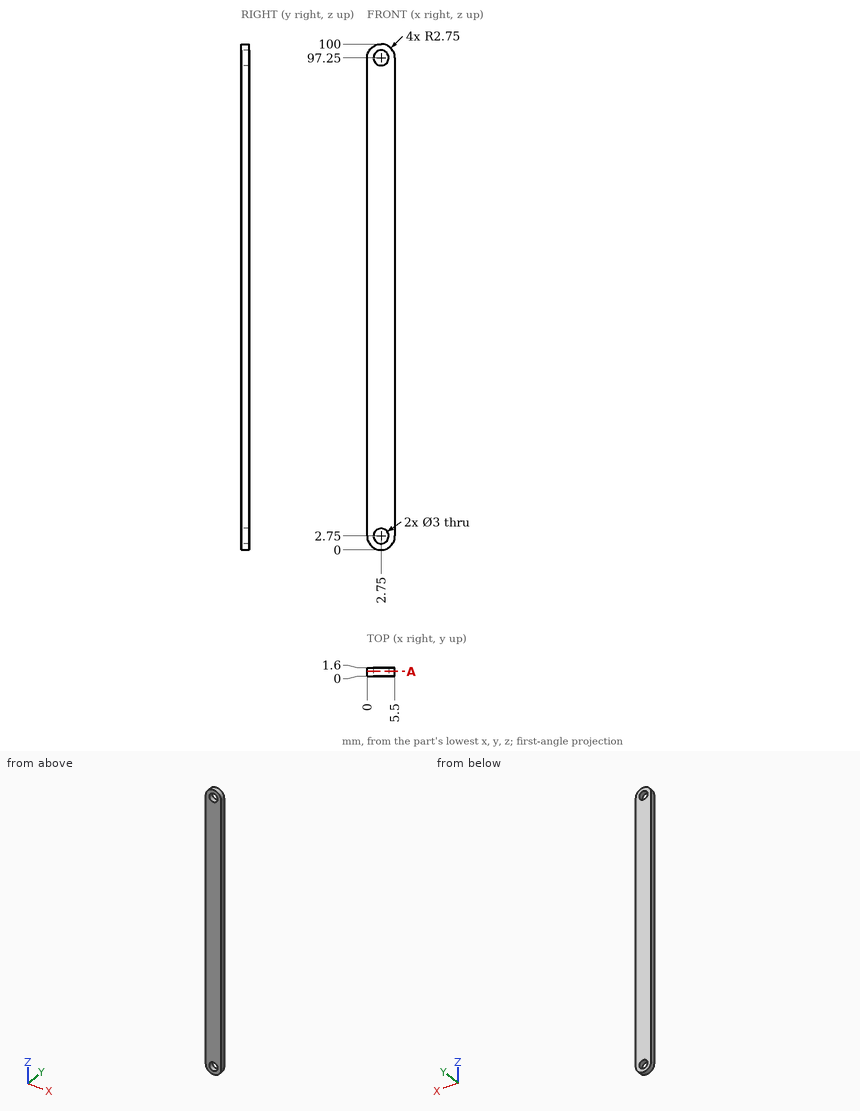
For this review, use the dimensioned drawing (mm, ordinates from the lowest corner) and the shaded views. Give positions to 0.01 mm unless a question says otherwise; leave off trailing zeros. Use one line per item in the form item = value. Start each with the question number.
Item 1: We need section A-A on y = 0.9. Give the number of separate pieces and of enclosed holes in the cut face, plus the area to 3 significant figures.
Item 2: Insertion check: pin 1 Ø2.5 at (x, z) = (2.75, 2.75) entering from -Y. The pin has a flat end and moves straight along its axis. Give the tip position at first contact, or say it passes through.
Item 3: To check wall thickness, follow line 1 along Z through (x, y) = (2.75, 1.1); line 2 along Z through (x, y) = (3.3, 1.15); line 3 along X through (y, z) = (1.2, 97.25). State the ranges of each line that lie inside material, in increasing order. Write a range as from..to.
Completed:
q1.separate_pieces = 1
q1.enclosed_holes = 2
q1.area = 529 mm²
q2.pin_1 = through
q3.line_1 = 0..1.25, 4.25..95.75, 98.75..100
q3.line_2 = 0.06..1.35, 4.15..95.85, 98.65..99.94
q3.line_3 = 0..1.25, 4.25..5.5
